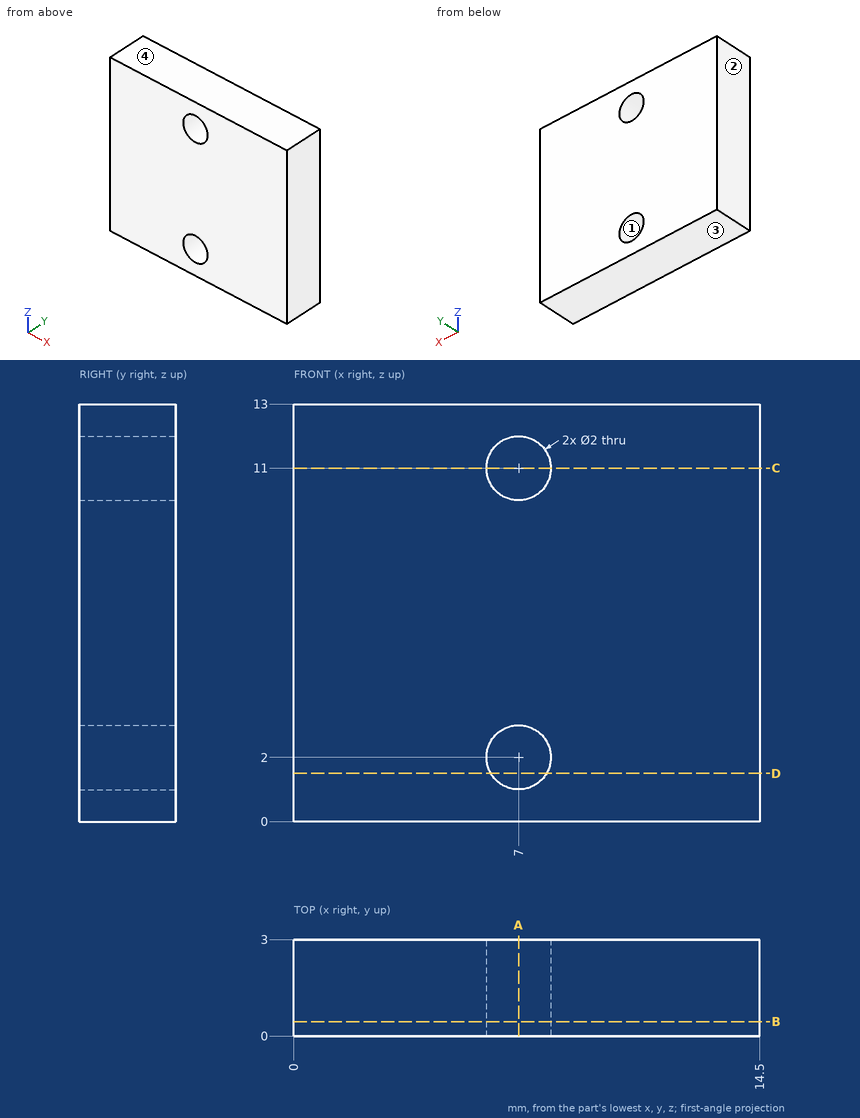
The drawing under review shows one solid part. Ordinate dimensions are in mm from its lowest x, y, z. Give positions to 0.01 mm unless a question says otherwise; leave off trailing zeros. Loops run counter-clockwise (first coordinate to the right, second up) from the corner with the lowest first, then second, coordinate; pieces in that order, holes last. Notation, with made-up numbers: M -0.5,18 L 47.5,18 A16 cw 47.5,49 Z; hole C -32.5,43 d1. An arc over 180 degrees is marked long. One line per item, written item: value. Start each with the question number.
Q1. Add section B-B (y = 0.45). Give the boundary of the cut face in (x, z), and give its area (3 significant figures).
Q2. Add section A-A (x = 7). Give the boundary of the cut face in (y, z), and give its area (3 significant figures).
Q3. For L1, parallel to Z at x = 7, y = 1.45; L2, parallel to X at y = 1.75, z = 11, list the stretches that pass through material, from the lowest coordinate up.
Q4. Draft analysis for pull direction Z (two halves, no side actions). For the marked faces 1, 2, 3 and 4, state which applies: released by +Z, released by -Z, zero draft, split by the parting line, or undercut.
Q5. Add section D-D (z = 1.5). Give the boundary of the cut face in (x, y), and give its area (3 significant figures).
Q6. Add section C-C (z = 11). Give the boundary of the cut face in (x, y), and give its area (3 significant figures).
Q7. Clearance check with a flat-ended pin moving along its axis: pin 1 Ø1.6 at (x, z) = (7, 2) entering from -Y. State where the tip first meets the part, or that it passes through.
Reply:
1. outline: M 0,0 L 14.5,0 L 14.5,13 L 0,13 Z; hole C 7,2 d2; hole C 7,11 d2
1. area: 182 mm²
2. outline: M 0,0 L 3,0 L 3,1 L 0,1 Z; M 0,3 L 3,3 L 3,10 L 0,10 Z; M 0,12 L 3,12 L 3,13 L 0,13 Z
2. area: 27.0 mm²
3. L1: 0 to 1, 3 to 10, 12 to 13
3. L2: 0 to 6, 8 to 14.5
4. face 1: undercut
4. face 2: zero draft
4. face 3: released by -Z
4. face 4: released by +Z
5. outline: M 0,0 L 6.13,0 L 6.13,3 L 0,3 Z; M 7.87,0 L 14.5,0 L 14.5,3 L 7.87,3 Z
5. area: 38.3 mm²
6. outline: M 0,0 L 6,0 L 6,3 L 0,3 Z; M 8,0 L 14.5,0 L 14.5,3 L 8,3 Z
6. area: 37.5 mm²
7. pin 1: through
